Verification items for the finished model (mm, model axes). A direction names the side the tool comes from. Coordinates: 2 decimals unless noted, no trailing zeros. Write each loop counter-clockwise with the first axis right and the second up, starting at its lowest first coordinate (ties: lowest second). Pieces come first, ordered by that corner, then holes. Notation, with made-up numbers: (-39, 41.5) -> (-19, 41.5) arc R20 ccw to (-19, 55.5) -> close; hole circle Ø7 at (-32.5, 56.5). An arc over 180 degrees is marked (long way). Use a Markdown table: item, result. Add a question column.
from build123d import *

# Parameters (mm, degrees)
SKETCH_R     = 1.850117
PAD_DEPTH    = 1.57
SKETCH001_W  = 20
SKETCH001_H  = 10
PAD001_DEPTH = 10


with BuildPart() as part:
    # Sketch → Pad (new body)
    with BuildSketch(Plane.XZ):
        Polygon((0, 0), (8.46819, 0), (8.46819, 4.940975), (24.558208, 4.940975), (24.558208, 0), (32.146711, 0), (32.146711, 4.940975), (35.739379, 4.940975), (35.739379, 0), (60.955266, 0), (60.955266, 4.940975), (64.547934, 4.940975), (64.547934, 0), (72.136436, 0), (72.136436, 4.940975), (84.565834, 4.940975), (84.565834, 22.469307), (0, 22.469307), align=None)
        with Locations((3.4028, 4.726487)):
            Circle(SKETCH_R, mode=Mode.SUBTRACT)
        with Locations((3.4028, 18.717941)):
            Circle(SKETCH_R, mode=Mode.SUBTRACT)
    extrude(amount=PAD_DEPTH)

    # Sketch001 (on Face22 of Pad) → Pad001 (join)
    with BuildSketch(Plane.XZ.offset(5.785)):
        with Locations((31.353824, 27.469307)):
            Rectangle(SKETCH001_W, SKETCH001_H)
    extrude(amount=-PAD001_DEPTH)


solid = part.part
1) Cross-section at A-A on x = 50.5. Record the boundary of the cut face in (y, z), then the cut area to 3 significant figures.
2) Gauge pin test, flat ends, axial feed: pin 1 (0.8 mm diameter, centred on y = -1, z = 3.5, fed in from +X); pin 2 (3 mm diameter, centred on x = 3.4, z = 18.72, fed in from +Y); pin 3 (1.3 mm diameter, centred on x = 31.5, y = 2.5, fed in from -Z); pin 4 (1.7 mm diameter, centred on y = -1, z = 2, fed in from -X). Record the tip position at first contact, or that the pin passes through.
3) Thickness scan on L1, parallel to Y at x = 55.5, z = 2; L2, parallel to Z at x = 40.5, y = -2.5; L3, parallel to X at y = -4, z = 26.5. Record the ranges inside material, lowest first.
4) Cross-section at B-B on y = -4.5. Record the boundary of the cut face in (x, z), then the cut area to 3 significant figures.
5) Set-up check for faces 5 (the face through (31, 2, 22.469)), 6 (the face through (60.955, -1, 2)), 7 (the face through (72.136, -1, 2)): record each of +Z, -Z, +X, -X, +Y, -Y from which the full face is reachable in a straight line by a thin tool's end or side.
6) Release check for a two-part mould opening along X. For faces 1 (the face through (21.354, -1, 27)), 2 (the face through (8.468, -1, 2)), 3 (the face through (42, -1.57, 11)), 4 (the face through (63, -1, 4.941)) record: released by +X, released by -X, zero draft, split by the parting line, or undercut.
Returned:
| question | item | result |
|---|---|---|
| 1 | outline | (-1.57, 0) -> (0, 0) -> (0, 22.47) -> (-1.57, 22.47) -> close |
| 1 | area | 35.3 mm² |
| 2 | pin 1 | stops at x = 72.14 |
| 2 | pin 2 | passes through |
| 2 | pin 3 | stops at z = 22.47 |
| 2 | pin 4 | stops at x = 0 |
| 3 | L1 | y = -1.57 to 0 |
| 3 | L2 | z = 22.47 to 32.47 |
| 3 | L3 | x = 21.35 to 41.35 |
| 4 | outline | (21.35, 22.47) -> (41.35, 22.47) -> (41.35, 32.47) -> (21.35, 32.47) -> close |
| 4 | area | 200 mm² |
| 5 | face 5 | -Z, +X, -X, +Y |
| 5 | face 6 | -Z, +Y, -Y |
| 5 | face 7 | -Z, +X, +Y, -Y |
| 6 | face 1 | released by -X |
| 6 | face 2 | undercut |
| 6 | face 3 | zero draft |
| 6 | face 4 | undercut |
